from build123d import *

# Parameters (mm, degrees)
SKETCH_1_R               = 50
EXTRUDE_1_DEPTH          = 57.7
SKETCH_2_W               = 88.552643685
SKETCH_2_H               = 15.944116671
SKETCH_2_W_2             = 133.424200465
SKETCH_2_H_2             = 21.693790907
CUT_EXTRUDE_1_DEPTH      = 57.7
SKETCH_3_W               = 51.791054301
SKETCH_3_H               = 91.732420586
SKETCH_3_W_2             = 35.451128289
SKETCH_3_H_2             = 96.304213357
CUT_EXTRUDE_2_DEPTH      = 40
CUT_EXTRUDE_3_DEPTH      = 35
CUT_EXTRUDE_3_DEPTH_BACK = 77
SKETCH_5_W               = 7.7
SKETCH_5_H               = 94.441631117


with BuildPart() as part:
    # 草图1 → 凸台-拉伸1 (new body)
    with BuildSketch(Plane.XY):
        Circle(SKETCH_1_R)
    extrude(amount=EXTRUDE_1_DEPTH)

    # 草图2 → 切除-拉伸1 (cut)
    with BuildSketch(Plane.XY.offset(57.7)):
        with Locations((0.613398072, 54.174358248)):
            Rectangle(SKETCH_2_W, SKETCH_2_H)
        with Locations((13.337614445, -57.096895454)):
            Rectangle(SKETCH_2_W_2, SKETCH_2_H_2)
    extrude(amount=-CUT_EXTRUDE_1_DEPTH, mode=Mode.SUBTRACT)

    # 草图3 → 切除-拉伸2 (cut)
    with BuildSketch(Plane(origin=(0, 0, 0), x_dir=(-1, 0, 0), z_dir=(0, 0, -1))):
        with Locations((-45.009592204, 0.336089619)):
            Rectangle(SKETCH_3_W, SKETCH_3_H)
        with Locations((36.839629198, -1.949806767)):
            Rectangle(SKETCH_3_W_2, SKETCH_3_H_2)
    extrude(amount=-CUT_EXTRUDE_2_DEPTH, mode=Mode.SUBTRACT)

    # 草图5 → 切除-拉伸3 (cut, two sides: drawn at the far end of the back side and taken through both)
    with BuildSketch(Plane.ZY.offset(19.114065053).offset(-CUT_EXTRUDE_3_DEPTH_BACK)):
        with Locations((53.85, -1.018515647)):
            Rectangle(SKETCH_5_W, SKETCH_5_H)
    extrude(amount=CUT_EXTRUDE_3_DEPTH + CUT_EXTRUDE_3_DEPTH_BACK, mode=Mode.SUBTRACT)


solid = part.part
Verification items for the finished model (mm, model axes). A direction names the side the tool comes from. Give positions to 0.01 mm unless a question says otherwise; leave off trailing zeros. Loops run counter-clockwise (first coordinate to the right, second up) from the corner with the lowest first, then second, coordinate; pieces in that order, holes last.
1. Cross-section at D-D on y = -29. Record the cut outline in (x, z).
Derived:
outline: (-40.73, 40) - (-19.11, 40) - (-19.11, 0) - (19.11, 0) - (19.11, 40) - (40.73, 40) - (40.73, 50) - (-40.73, 50) - close
2. Cross-section at A-A on y = 14. Record the cut outline in (x, z).
Derived:
outline: (-48, 40) - (-19.11, 40) - (-19.11, 0) - (19.11, 0) - (19.11, 40) - (48, 40) - (48, 50) - (-48, 50) - close
3. Material ranges on probe 1 along X at (y, z) = (40, 29.5); probe 2 along Z at (x, y) = (23, -26); probe 3 along Y at (x, z) = (-28, 44), recorded low to high.
Derived:
probe 1: x = -19.11 to 19.11
probe 2: z = 40 to 50
probe 3: y = -41.42 to 41.42
4. Tool access check on faces 1 (the cylindrical face through (-50, 0, 45)), 2 (the flat face through (-19.114, -1, 20)), 3 (the flat face through (19.114, 0, 20)). Record the directions out of +Z, -Z, +X, -X, +Y, -Y that give a thin tool (end or side, any length) a straight path to the whole face; none if there is none.
Derived:
face 1: +Z, -Z, -X
face 2: -Z, -X, +Y, -Y
face 3: -Z, +X, +Y
5. Cross-section at B-B on z = 6.5. Record the cut outline in (x, y), and give its area (3 significant figures).
Derived:
outline: (-19.11, -46.2) arc R50 ccw to (-19, -46.25) - (19, -46.25) arc R50 ccw to (20.66, -45.53) - (19.11, -45.53) - (19.11, 46.2) - (-19.11, 46.2) - close
area: 3,530 mm2
6. Cross-section at C-C on x = 34. Record the cut outline in (y, z).
Derived:
outline: (-36.66, 40) - (36.66, 40) - (36.66, 50) - (-36.66, 50) - close
7. Go/stop test with flat-tipped pins: P1, Ø10, axis at x = -28.5, y = 33.5, coming from the -Z side; P2, Ø2, axis at y = 23, z = 25.5, coming from the +X side; P3, Ø1.2, axis at x = 20, z = 13.5, coming from the +Y side; P4, Ø12, axis at x = 20.5, z = 13, coming from the -Y side. Record where each tip stops, or that it passes through.
Derived:
P1: stops at z = 40
P2: stops at x = 19.11
P3: stops at y = -45.53
P4: stops at y = -46.25
